from build123d import *

# Parameters (mm, degrees)
BOSS_EXTRUDE1_DEPTH   = 2
CHAMFER1_SIZE         = 10
CHAMFER2_SIZE         = 35
FILLET1_R             = 10
F_5_0MM_DOWEL_HOLE1_D = 5
SKETCH5_R             = 2.5
CUT_EXTRUDE2_DEPTH    = 280.543377672
CUT_EXTRUDE3_DEPTH    = 280.543377672


with BuildPart() as part:
    # Sketch1 → Boss-Extrude1 (new body)
    with BuildSketch(Plane(origin=(0, 0, 0), x_dir=(1, 0, 0), z_dir=(0, 1, 0))):
        Polygon((56, 56), (129.5, 70.5), (270.5, 70.5), (270.5, -70.5), (129.5, -70.5), (56, -56), (-56, -56), (-56, 56), align=None)
    extrude(amount=BOSS_EXTRUDE1_DEPTH)

    # Chamfer1
    chamfer1_edges = [part.edges().sort_by_distance(p)[0] for p in [
        (-56, 1, 56),
        (-56, 1, -56),
    ]]
    chamfer(chamfer1_edges, length=CHAMFER1_SIZE)

    # Chamfer2
    chamfer2_edges = [part.edges().sort_by_distance(p)[0] for p in [
        (270.5, 1, 70.5),
        (270.5, 1, -70.5),
    ]]
    chamfer(chamfer2_edges, length=CHAMFER2_SIZE)

    # Fillet1
    fillet1_edges = [part.edges().sort_by_distance(p)[0] for p in [
        (129.5, 1, 70.5),
        (56, 1, 56),
        (56, 1, -56),
        (129.5, 1, -70.5),
        (-56, 1, 46),
        (-56, 1, -46),
        (-46, 1, -56),
        (-46, 1, 56),
        (235.5, 1, -70.5),
        (270.5, 1, 35.5),
        (270.5, 1, -35.5),
        (235.5, 1, 70.5),
    ]]
    fillet(fillet1_edges, radius=FILLET1_R)

    # Ø5.0mm Dowel Hole1 (through all)
    with Locations(Plane(origin=(0, 0, 0), x_dir=(-1, 0, 0), z_dir=(0, -1, 0))):
        with Locations((36, -36), (-36, -36), (36, 36), (-36, 36)):
            Hole(F_5_0MM_DOWEL_HOLE1_D / 2)

    # Sketch5 → Cut-Extrude2 (cut, through all)
    with BuildSketch(Plane(origin=(0, 2, 0), x_dir=(1, 0, 0), z_dir=(0, 1, 0))):
        with Locations(Location((200, 0, 0), (0, 0, 270))):
            Circle(SKETCH5_R)
    extrude(amount=-CUT_EXTRUDE2_DEPTH, mode=Mode.SUBTRACT)

    # Sketch6 → Cut-Extrude3 (cut, through all)
    with BuildSketch(Plane(origin=(0, 2, 0), x_dir=(1, 0, 0), z_dir=(0, 1, 0))):
        with BuildLine():
            Line((93.2, 20.5), (93.2, 49.5))
            ThreePointArc((93.2, 49.5), (93.053553391, 49.853553391), (92.7, 50))
            Line((92.7, 50), (90.5, 50))
            ThreePointArc((90.5, 50), (90.146446609, 49.853553391), (90, 49.5))
            Line((90, 49.5), (90, 20.5))
            ThreePointArc((90, 20.5), (90.146446609, 20.146446609), (90.5, 20))
            Line((90.5, 20), (92.7, 20))
            ThreePointArc((92.7, 20), (93.053553391, 20.146446609), (93.2, 20.5))
        make_face()
        with BuildLine():
            Line((90.5, -20), (92.7, -20))
            ThreePointArc((92.7, -20), (93.053553391, -20.146446609), (93.2, -20.5))
            Line((93.2, -20.5), (93.2, -49.5))
            ThreePointArc((93.2, -49.5), (93.053553391, -49.853553391), (92.7, -50))
            Line((92.7, -50), (90.5, -50))
            ThreePointArc((90.5, -50), (90.146446609, -49.853553391), (90, -49.5))
            Line((90, -49.5), (90, -20.5))
            ThreePointArc((90, -20.5), (90.146446609, -20.146446609), (90.5, -20))
        make_face()
    extrude(amount=-CUT_EXTRUDE3_DEPTH, mode=Mode.SUBTRACT)


solid = part.part
Part model, mm, in its own coordinate system. Round coordinates to 2 decimals unless told otherwise and drop trailing zeros. Write each loop counter-clockwise with the first axis right and the second up, starting at its lowest first coordinate (ties: lowest second). Pieces come first, ordered by that corner, then holes. Notation, with made-up numbers: M 38,-22.75 L 88,-22.75 A29 cw 88,3.25 Z; hole C 27.25,-25.75 d7. An arc over 180 degrees is marked long. Return JSON: item names as keys, results as strings. Group by question number.
(1) Saw through at B-B on x = 42.5. Write the cut outline in (y, z), then the cut area to 3 significant figures.
(2) Drill centre lines: probe 1 along Z at (x, y) = (-36, 0.55); probe 2 along X at (y, z) = (0.5, 36); probe 3 along X at (y, z) = (1.5, 0). Where is each one in solid material? Low to high.
(3) Pin check, flat tips, straight feed: pin 1 Ø8 at (x, z) = (212, 1.5) entering from -Y; pin 2 Ø1 at (x, y) = (92, 1) entering from +Z; pin 3 Ø0.6 at (y, z) = (1, -40.5) entering from +X; pin 4 Ø1 at (x, y) = (55.5, 0) entering from -Z. Stop position of each tip, or through.
(4) Saw through at A-A on y = 0.5. Count the separate pieces of the cut face and the enclosed holes in it, then the cut area to 3 significant figures.
(5) Saw through at C-C on z = -60.5. Write the cut outline in (x, y).
Returned:
{
 "1": {"outline": "M 0,-56 L 2,-56 L 2,56 L 0,56 Z", "area": "224 mm²"},
 "2": {"probe 1": "-56 to -38.5, -33.5 to 33.5, 38.5 to 56", "probe 2": "-56 to -38.5, -33.5 to 33.5, 38.5 to 90, 93.2 to 269.36", "probe 3": "-56 to 197.5, 202.5 to 270.5"},
 "3": {"pin 1": "y = 0", "pin 2": "z = 63.2", "pin 3": "x = 265.8", "pin 4": "z = -56.05"},
 "4": {"separate pieces": "1", "enclosed holes": "7", "area": "40,100 mm²"},
 "5": {"outline": "M 78.81,0 L 245.5,0 L 245.5,2 L 78.81,2 Z"}
}
